Geometry check sheet. Reference: the model listing, model coordinates, mm. Face numbers are marked on the shaded views. A direction names the side the tool comes from. Give positions to 0.01 mm unless a question says otherwise; leave off trailing zeros. Loops run counter-clockwise (first coordinate to the right, second up) from the corner with the lowest first, then second, coordinate; pieces in that order, holes last. Notation, with made-up numbers: (44, 78.25) -> (48, 78.25) arc R22 cw to (48, 92.25) -> close; hole circle Ø4 at (2, -11.75). An arc over 180 degrees is marked (long way). One line per question, with ' | ' between items.
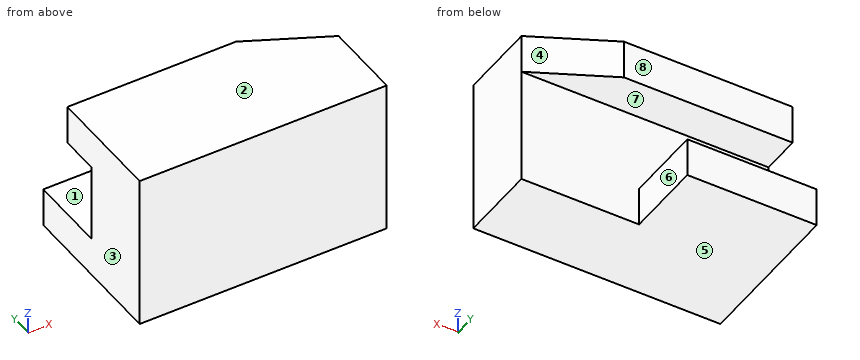
from build123d import *

# Parameters (mm, degrees)
BOSS_EXTRUDE1_DEPTH     = 20
SKETCH1_3_W             = 63
SKETCH1_3_H             = 10
BOSS_EXTRUDE2_DEPTH     = 30
SKETCH1_4_W             = 33
SKETCH1_4_H             = 10
BOSS_EXTRUDE3_DEPTH     = 40
CUT_EXTRUDE1_DEPTH      = 31
CUT_EXTRUDE1_DEPTH_BACK = 10


with BuildPart() as part:
    # Sketch1 → Boss-Extrude1 (new body)
    with BuildSketch(Plane(origin=(0, 0, 0), x_dir=(1, 0, 0), z_dir=(0, 1, 0))):
        Polygon((33, 30), (0, 30), (0, 10), (63, 10), (63, 40), (33, 40), align=None)
    extrude(amount=BOSS_EXTRUDE1_DEPTH)

    # Sketch1<3> → Boss-Extrude2 (add)
    with BuildSketch(Plane(origin=(0, 0, 0), x_dir=(1, 0, 0), z_dir=(0, 1, 0))):
        with Locations((31.5, 5)):
            Rectangle(SKETCH1_3_W, SKETCH1_3_H)
    extrude(amount=BOSS_EXTRUDE2_DEPTH)

    # Sketch1<4> → Boss-Extrude3 (add)
    with BuildSketch(Plane(origin=(0, 0, 0), x_dir=(1, 0, 0), z_dir=(0, 1, 0))):
        with Locations((16.5, 35)):
            Rectangle(SKETCH1_4_W, SKETCH1_4_H)
    extrude(amount=BOSS_EXTRUDE3_DEPTH)

    # Sketch2 → Cut-Extrude1 (cut, two sides)
    with BuildSketch(Plane(origin=(0, 0, -10), x_dir=(-1, 0, 0), z_dir=(0, 0, -1))) as cut_extrude1_sk:
        Polygon((-63, 30), (-63, 20), (-43, 30), align=None)
    extrude(amount=CUT_EXTRUDE1_DEPTH, mode=Mode.SUBTRACT)
    extrude(cut_extrude1_sk.sketch, amount=-CUT_EXTRUDE1_DEPTH_BACK, mode=Mode.SUBTRACT)


solid = part.part
Item 1: Sectioned sample at A-A (y = 25). Record the cut outline in (x, z), plus the area to 3 significant figures.
Result:
outline: (0, -40) -> (33, -40) -> (33, -30) -> (0, -30) -> close; (0, -10) -> (53, -10) -> (53, 0) -> (0, 0) -> close | area: 860 mm2
Item 2: Depth check by flat-ended pin: pin 1 Ø1.5 at (x, y) = (37, 32) entering from -Z; pin 2 Ø11 at (x, z) = (21.5, -6) entering from +Y; pin 3 Ø3 at (y, z) = (25.5, -32.5) entering from +X; pin 4 Ø3 at (x, z) = (14, -15.5) entering from +Y. Enter the tip coordinate at first touch or a pass-through.
Result:
pin 1: through | pin 2: y = 30 | pin 3: x = 33 | pin 4: y = 20
Item 3: Scan lines: probe 1 along Z at (x, y) = (4, 28.5); probe 2 along Y at (x, z) = (27, -11); probe 3 along Y at (x, z) = (19, -9.5). Record each from-to range of solid material in increasing order.
Result:
probe 1: -40 to -30, -10 to 0 | probe 2: 0 to 20 | probe 3: 0 to 30
Item 4: Sectioned sample at D-D (x = 55.5). Record the cut outline in (y, z), plus the area to 4 significant figures.
Result:
outline: (0, -40) -> (20, -40) -> (20, -10) -> (23.75, -10) -> (23.75, 0) -> (0, 0) -> close | area: 837.5 mm2
Item 5: Sectioned sample at C-C (z = -32). Record the cut outline in (x, y), plus the area to 3 significant figures.
Result:
outline: (0, 0) -> (63, 0) -> (63, 20) -> (33, 20) -> (33, 40) -> (0, 40) -> close | area: 1,920 mm2
Item 6: Release check for a two-part mould opening along Z. For the marked faces 1, 2 and 3 record: pulls with the +Z half, pulls with the -Z half, needs draft (parallel to the pull), parting line crosses it, or undercut.
Result:
face 1: undercut | face 2: pulls with the +Z half | face 3: needs draft
Item 7: Sectioned sample at B-B (x = 20). Record the cut outline in (y, z).
Result:
outline: (0, -40) -> (40, -40) -> (40, -30) -> (20, -30) -> (20, -10) -> (30, -10) -> (30, 0) -> (0, 0) -> close
Item 8: Set-up check for the marked faces 4, 5, 6, 7 and 8: record each of +Z, -Z, +X, -X, +Y, -Y from which the full face is reachable in a straight line by a thin tool's end or side.
Result:
face 4: +Z, -Z, +X, +Y | face 5: -Z, +X, -X, +Y, -Y | face 6: -Z, +X, +Y | face 7: +X, -X, +Y | face 8: +Z, +X, -X, +Y
